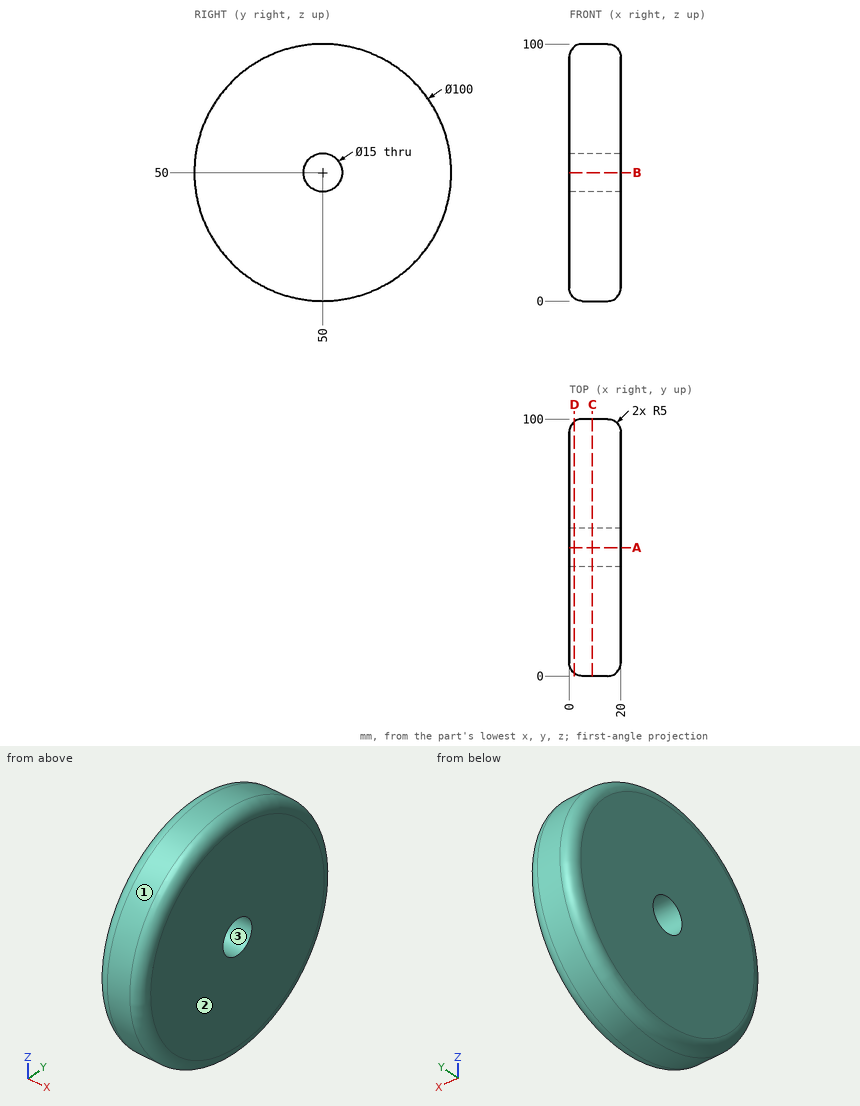
Job drawing, mm, ordinate dimensions from the low corner. One solid piece. Coordinates: 2 decimals unless noted, no trailing zeros. Write each loop counter-clockwise with the first axis right and the second up, starting at its lowest first coordinate (ties: lowest second). Pieces come first, ordered by that corner, then holes.
Item 1: Probe line 1 (Y direction, x = 11.5, z = 50); line 2 (Y direction, x = 4, z = 50); line 3 (Z direction, x = 2, y = 32.5). List the from-to ranges inside material, lowest first.
Item 2: Mould opens along Y. For the marked faces 1, 2 and 3 say: released by +Y, released by -Y, zero draft, split by the parting line, or undercut.
Item 3: Slice it at C-C (x = 9). Write the cut outline in (y, z).
Item 4: Slice it at D-D (x = 2). Write the cut outline in (y, z), and give its area (3 significant figures).
Item 5: Pin check, flat tips, straight feed: pin 1 (3 mm diameter, centred on x = 14, z = 24.5, fed in from -Y); pin 2 (10 mm diameter, centred on x = 15.5, z = 16.5, fed in from +Y); pin 3 (2 mm diameter, centred on x = 2.5, y = 34.5, fed in from +Z). Stop position of each tip, or through.
Item 6: Slice it at A-A (y = 50). Write the cut outline in (x, z).
Results found:
1. line 1: y = 0 to 42.5, 57.5 to 100
1. line 2: y = 0.1 to 42.5, 57.5 to 99.9
1. line 3: z = 4.23 to 95.77
2. face 1: split by the parting line
2. face 2: zero draft
2. face 3: undercut
3. outline: circle Ø100 at (50, 50); hole circle Ø15 at (50, 50)
4. outline: circle Ø98 at (50, 50); hole circle Ø15 at (50, 50)
4. area: 7,370 mm2
5. pin 1: stops at y = 6.14
5. pin 2: stops at y = 91.07
5. pin 3: stops at z = 97.42
6. outline: (0, 5) arc R5 ccw to (5, 0) - (15, 0) arc R5 ccw to (20, 5) - (20, 42.5) - (0, 42.5) - close; (0, 57.5) - (20, 57.5) - (20, 95) arc R5 ccw to (15, 100) - (5, 100) arc R5 ccw to (0, 95) - close
